```python
from build123d import *

# Parameters (mm, degrees)
SKETCH1_R           = 1.5
BOSS_EXTRUDE1_DEPTH = 4
FILLET1_R           = 5


with BuildPart() as part:
    # Sketch1 → Boss-Extrude1 (new body)
    with BuildSketch(Plane.XY):
        with BuildLine():
            Line((-20.616075737, 20.616075737), (-63.042482608, -21.810331134))
            ThreePointArc((-63.042482608, -21.810331134), (-64.214055483, -24.638758259), (-63.042482608, -27.467185384))
            add(Edge.make_bspline(
                [(-63.042482608, -27.467185384), (-44.475149979, -46.28503097), (-11.38960692, -52.316770126), (5.656854249, -35.575297224)],
                knots=[0, 0, 0, 0, 1, 1, 1, 1], degree=3))
            Line((5.656854249, -35.575297224), (8.485658906, -32.746492568))
            Line((8.485658906, -32.746492568), (32.746492568, -8.485658906))
            Line((32.746492568, -8.485658906), (35.575297224, -5.656854249))
            ThreePointArc((35.575297224, -5.656854249), (37.918442975, 0), (35.575297224, 5.656854249))
            Line((35.575297224, 5.656854249), (5.680184525, 35.551966949))
            ThreePointArc((5.680184525, 35.551966949), (0.032993992, 37.918442975), (-5.633523974, 35.5986275))
            Line((-5.633523974, 35.5986275), (-20.616075737, 20.616075737))
        make_face()
        with Locations((29.918065443, -5.657231781)):
            Circle(SKETCH1_R, mode=Mode.SUBTRACT)
        with Locations((5.657231781, -29.918065443)):
            Circle(SKETCH1_R, mode=Mode.SUBTRACT)
        with Locations((-17.787648612, 17.787648612)):
            Circle(SKETCH1_R, mode=Mode.SUBTRACT)
        with Locations((-60.214055483, -24.638758259)):
            Circle(SKETCH1_R, mode=Mode.SUBTRACT)
        Polygon((29.918442975, 0), (0, -29.918442975), (-29.918442975, 0), (-14.959221487, 14.959221487), (0, 29.918442975), align=None, mode=Mode.SUBTRACT)
    extrude(amount=BOSS_EXTRUDE1_DEPTH)

    # Fillet1
    fillet1_edges = [part.edges().sort_by_distance(p)[0] for p in [
        (-29.918442975, 0, 2),
        (0, -29.918442975, 2),
        (29.918442975, 0, 2),
        (0, 29.918442975, 2),
    ]]
    fillet(fillet1_edges, radius=FILLET1_R)


solid = part.part
```
The model under review builds one solid part; all positions refer to its coordinate system, in mm. A direction names the side the tool comes from. Round coordinates to 2 decimals unless told otherwise and drop trailing zeros. Write each loop counter-clockwise with the first axis right and the second up, starting at its lowest first coordinate (ties: lowest second). Pieces come first, ordered by that corner, then holes. Notation, with made-up numbers: (-40, -10.75) - (-20, -10.75) arc R18 cw to (-20, 4.25) - close; hole circle Ø10 at (55, -31). An arc over 180 degrees is marked (long way). One line per question, with ' | ' between items.
Item 1: To check wall thickness, follow probe 1 along X at (y, z) = (-5.5, 3.15); probe 2 along Y at (x, z) = (-19, 2.7); probe 3 along Y at (x, z) = (-22, 1.2). State the ranges of each line that lie inside material, in increasing order.
Resolved:
probe 1: x = -46.73 to -24.42, 24.42 to 28.43, 31.41 to 35.73 | probe 2: y = -45.34 to -10.92, 10.92 to 16.9, 18.67 to 22.23 | probe 3: y = -45.36 to -7.92, 7.92 to 19.23
Item 2: For P1, Ø2, axis at y = -3.5, z = 2, coming from the -X side; P2, Ø1, axis at y = 2, z = 2, coming from the -X side, all flat-tipped, find the tip position at first contact; note any pin that passes through.
Resolved:
P1: stops at x = -45.73 | P2: stops at x = -39.73
Item 3: Add section B-B, the plane y = -17. Give the boundary of the cut face in (x, z).
Resolved:
outline: (-58.23, 0) - (-12.92, 0) - (-12.92, 4) - (-58.23, 4) - close; (12.92, 0) - (24.23, 0) - (24.23, 4) - (12.92, 4) - close
Item 4: Add section C-C, the plane z = 1.4. State how many separate pieces and enclosed holes the cut face has, then the cut area to 3 significant figures.
Resolved:
separate pieces: 1 | enclosed holes: 5 | area: 3,080 mm2
Item 5: The part is to be moulded in two halves that separate along Y. For faces 1 (the face through (14.8, 15.12, 1.97)), 2 (the face through (-33.936, 7.296, 1.972)), 3 (the face through (-64.214, -24.595, 1.972)), say which applies: pulls with the +Y half, pulls with the -Y half, needs draft (parallel to the pull), parting line crosses it, or undercut.
Resolved:
face 1: undercut | face 2: pulls with the +Y half | face 3: parting line crosses it
Item 6: Add section A-A, the plane x = 24.5. Give the boundary of the cut face in (y, z), then the cut area to 3 significant figures.
Resolved:
outline: (-16.73, 0) - (-5.42, 0) - (-5.42, 4) - (-16.73, 4) - close; (5.42, 0) - (16.73, 0) - (16.73, 4) - (5.42, 4) - close | area: 90.5 mm2
Item 7: For faces 4 (the face through (-27.847, 0.055, 2.028)), 5 (the face through (-21, -14, 0)), list the 3-axis set-ups (+Z, -Z, +X, -X, +Y, -Y) from which the entire face can be reached by the end or side of a thin tool; tool diameter is ignored.
Resolved:
face 4: +Z, -Z | face 5: -Z, +X, -X, +Y, -Y
